Can you work these out from the model? Positions are in its coordinate system, mm. Face numbers are marked on the shaded views. A direction names the side the tool comes from. Coordinates: 2 decimals unless noted, no trailing zeros. Loops run counter-clockwise (first coordinate to the right, second up) from the corner with the lowest first, then second, coordinate; pieces in that order, holes last.
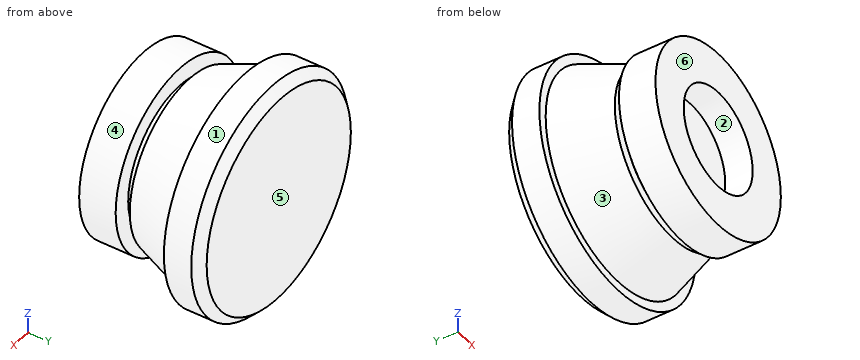
```python
from build123d import *

# Parameters (mm, degrees)
SKETCH3_R          = 5.5
CUT_EXTRUDE1_DEPTH = 3


with BuildPart() as part:
    # Sketch2 → Revolve1 (revolve)
    with BuildSketch(Plane.XY):
        Polygon((0, 0), (0, 15), (11.5, 15), (12.5, 14), (12.5, 11), (11.5, 11), (9.202672606, 5), (8, 5), (8, 4), (10, 4), (10, 0), align=None)
    revolve(axis=Axis((0, 15.75, 0), (0, -1, 0)))

    # Sketch3 → Cut-Extrude1 (cut)
    with BuildSketch(Plane.XZ):
        Circle(SKETCH3_R)
    extrude(amount=-CUT_EXTRUDE1_DEPTH, mode=Mode.SUBTRACT)


solid = part.part
```
(1) I want a section at C-C on y = 13.5. Write out the boundary of the cut face in (x, z), then the cut area to 3 significant figures.
Check values:
outline: circle Ø25 at (0, 0)
area: 491 mm2
(2) Which directions (+Z, -Z, +X, -X, +Y, -Y) give clear straight access to the entire face, cutting with the end or side of a thin tool? Please do the marked faces 1 and 2.
Check values:
face 1: +Y, -Y
face 2: -Y
(3) If I drill on probe 1 along Y at (x, z) = (8.25, -0.25); probe 2 along Z at (x, y) = (0, 1.6); probe 3 along Y at (x, z) = (-7.75, 5.5), over which ranges is the centre line in solid material (lowest first)?
Check values:
probe 1: y = 0 to 4, 5 to 15
probe 2: z = -10 to -5.5, 5.5 to 10
probe 3: y = 0 to 4, 5.79 to 15
(4) I want a section at B-B on z = 0. Write out the boundary of the cut face in (x, y).
Check values:
outline: (-12.5, 11) - (-11.5, 11) - (-9.2, 5) - (-8, 5) - (-8, 4) - (-10, 4) - (-10, 0) - (-5.5, 0) - (-5.5, 3) - (5.5, 3) - (5.5, 0) - (10, 0) - (10, 4) - (8, 4) - (8, 5) - (9.2, 5) - (11.5, 11) - (12.5, 11) - (12.5, 14) - (11.5, 15) - (-11.5, 15) - (-12.5, 14) - close
(5) I want a section at A-A on x = 0. Write out the boundary of the cut face in (y, z), then the cut area to 3 significant figures.
Check values:
outline: (0, -10) - (4, -10) - (4, -8) - (5, -8) - (5, -9.2) - (11, -11.5) - (11, -12.5) - (14, -12.5) - (15, -11.5) - (15, 11.5) - (14, 12.5) - (11, 12.5) - (11, 11.5) - (5, 9.2) - (5, 8) - (4, 8) - (4, 10) - (0, 10) - (0, 5.5) - (3, 5.5) - (3, -5.5) - (0, -5.5) - close
area: 286 mm2
(6) I'm going to push flat-ended pins straight in: pin 1 (1.5 mm diameter, centred on x = -7, y = 12, fed in from +Z); pin 2 (8 mm diameter, centred on x = 4.5, y = 4.5, fed in from -Z); pin 3 (4 mm diameter, centred on y = 12, z = 2.5, fed in from -X). Where does each tip first touch, or does it pass through?
Check values:
pin 1: stops at z = 10.83
pin 2: stops at z = -10.03
pin 3: stops at x = -12.49
(7) If we mould it in two halves opening along Y, with no side actions, what happens to the marked faces 3, 4, 5 and 6? For each: released by +Y, released by -Y, zero draft, split by the parting line, or undercut.
Check values:
face 3: undercut
face 4: zero draft
face 5: released by +Y
face 6: released by -Y
